from build123d import *

# Parameters (mm, degrees)
ESQUISSE1_W        = 100
ESQUISSE1_H        = 40
BOSS_EXTRU_1_DEPTH = 2
ESQUISSE3_W        = 5
ESQUISSE3_H        = 22
BOSS_EXTRU_2_DEPTH = 20
ESQUISSE4_W        = 8
ESQUISSE4_H        = 3
BOSS_EXTRU_3_DEPTH = 35


with BuildPart() as part:
    # Esquisse1 → Boss.-Extru.1 (new body)
    with BuildSketch(Plane.XY):
        Rectangle(ESQUISSE1_W, ESQUISSE1_H)
    extrude(amount=BOSS_EXTRU_1_DEPTH)

    # Esquisse3 → Boss.-Extru.2 (add)
    with BuildSketch(Plane.XY.offset(2)):
        with Locations((-35.5, -2)):
            Rectangle(ESQUISSE3_W, ESQUISSE3_H)
    extrude(amount=BOSS_EXTRU_2_DEPTH)

    # Esquisse4 → Boss.-Extru.3 (add)
    with BuildSketch(Plane.XY):
        with Locations((42, -14.5)):
            Rectangle(ESQUISSE4_W, ESQUISSE4_H)
    extrude(amount=BOSS_EXTRU_3_DEPTH)


solid = part.part
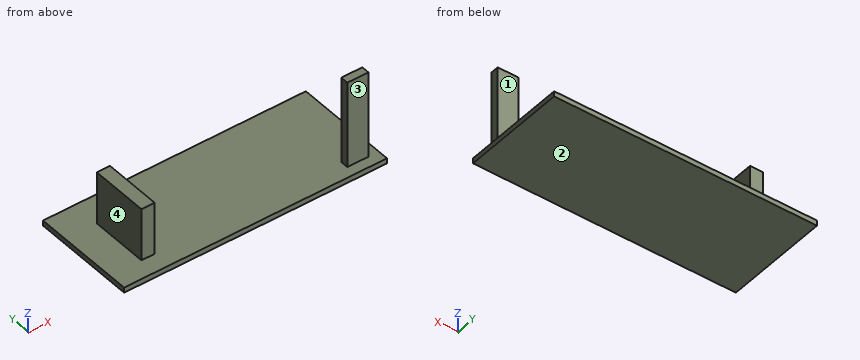
Work out the finished part from the listing and answer in its coordinate system (mm). Face numbers are marked on the shaded views. A direction names the side the tool comes from. Give positions to 0.01 mm unless a question says otherwise; leave off trailing zeros. Write each loop counter-clockwise with the first axis right and the second up, starting at its lowest first coordinate (ties: lowest second). Pieces come first, ordered by that corner, then holes. Notation, with made-up numbers: M -2.5,58.25 L 17.5,58.25 A23 ccw 17.5,87.25 Z; hole C 39,3.25 d2. An arc over 180 degrees is marked long. Answer as CSV lines item,"result".
Q1. A cutting plane is placed at D-D on z = 26. Write down the section's boundary in (x, y).
A:
outline,"M 38,-16 L 46,-16 L 46,-13 L 38,-13 Z"
Q2. A cutting plane is placed at C-C on y = -14. Write down the section's boundary in (x, z), plus the area to 3 significant figures.
A:
outline,"M -50,0 L 50,0 L 50,2 L 46,2 L 46,35 L 38,35 L 38,2 L -50,2 Z"
area,"464 mm²"
Q3. A tool of negligible diameter and unlimited length cuts with its end or side. For the marked faces 1, 2, 3 and 4, from which of +Z, -Z, +X, -X, +Y, -Y can it reach the whole face along a straight path? Write none if from no direction.
A:
face 1,"+Z, +X, +Y"
face 2,"-Z, +X, -X, +Y, -Y"
face 3,"+Z, +X, -X, -Y"
face 4,"+Z, -X, +Y, -Y"
Q4. Given P1, Ø6, axis at y = 9.5, z = 7.5, coming from the -X side; P2, Ø12, axis at x = -17, y = 2, coming from the +Z side; P3, Ø2, axis at y = 11.5, z = 9, coming from the -X side; P4, Ø6, axis at y = -7, z = 12.5, coming from the +X side, each flat-ended and moving along its own axis, determine where each tip first touches the part or whether it passes through.
A:
P1,"stops at x = -38"
P2,"stops at z = 2"
P3,"passes through"
P4,"stops at x = -33"
Q5. A cutting plane is placed at A-A on z = 7. Write down the section's boundary in (x, y), plus the area to 3 significant figures.
A:
outline,"M -38,-13 L -33,-13 L -33,9 L -38,9 Z; M 38,-16 L 46,-16 L 46,-13 L 38,-13 Z"
area,"134 mm²"
Q6. A cutting plane is placed at B-B on x = 42. Write down the section's boundary in (y, z).
A:
outline,"M -20,0 L 20,0 L 20,2 L -13,2 L -13,35 L -16,35 L -16,2 L -20,2 Z"
Q7. Find the intervals of material crossed by probe 1 along X at (y, z) = (1, 3); probe 2 along Z at (x, y) = (12, 1), in increasing order. Write a range as [from, to].
A:
probe 1,"x = [-38, -33]"
probe 2,"z = [0, 2]"
